Check sheet for the modelled part. Datum: model origin and axes. Units: mm. A direction names the side the tool comes from. Give positions to 0.01 mm unless a question says otherwise; leave off trailing zeros. Loops run counter-clockwise (first coordinate to the right, second up) from the corner with the lowest first, then second, coordinate; pieces in that order, holes last. Notation, with made-up numbers: (47.5, 45) -> (63.5, 45) arc R29 cw to (63.5, 82) -> close; hole circle Ø2 at (-19.5, -28.5). An arc over 180 degrees is marked (long way). Write each question's results on one line, items separated by ' | '. Start each with the question number.
Item 1: Cross-section at D-D on x = -2.5. Enter the section's corners in (y, z), then the cut area to 3 significant figures.
Item 2: Cross-section at A-A on z = 65.5. Enter the section's corners in (x, y).
Item 3: Cross-section at B-B on x = 12.5. Enter the section's corners in (y, z), then the cut area to 3 significant figures.
Item 4: Mould release check, pull along X, two halves, no side actions. Record for faces 1 (the face through (12, -2, 0)), 2 (the face through (10.476, -1.972, 8.448)), 3 (the face through (-16.07, -1.97, 54.5)), 4 (the face through (24, -2, 96)): pulls with the +X half, pulls with the -X half, needs draft (parallel to the pull), parting line crosses it, or undercut.
Item 5: Cross-section at C-C on y = -0.6. Enter the section's corners in (x, z), then the cut area to 3 significant figures.
Item 6: Gauge pin test, flat ends, axial feed: pin 1 Ø6 at (x, z) = (12.5, 10) entering from -Y; pin 2 Ø1 at (y, z) = (-2.5, 29) entering from +X. Record the tip position at first contact, or that the pin passes through.
Item 7: Scan lines: line 1 along Z through (x, y) = (12.5, -2.45); line 2 along X through (y, z) = (-2.8, 67.5); line 3 along Z through (x, y) = (-5.5, -2.6). Record each from-to range of solid material in increasing order.
Item 8: Access from +Z, -Z, +X, -X, +Y, -Y to the whole of each face (thin tool, end or side, straight path). Record for faces 5 (the face through (3, -4, 61)), 6 (the face through (0, -2, 27)).
from build123d import *

# Parameters (mm, degrees)
F0_R     = 2.55
F0_R_2   = 4
F1_DEPTH = 4


with BuildPart() as f1:
    # F0 (on Front) → F1 (new body)
    with BuildSketch(Plane.XZ):
        with BuildLine():
            Line((0, 48), (0, 5))
            ThreePointArc((0, 5), (1.464466, 1.464466), (5, 0))
            Line((5, 0), (20, 0))
            ThreePointArc((20, 0), (21.81842, 0.342388), (23.387798, 1.322661))
            ThreePointArc((23.387798, 1.322661), (16.523699, 23.80604), (25, 45.73252))
            Line((25, 45.73252), (25, 93))
            ThreePointArc((25, 93), (23.535534, 96.535534), (20, 98))
            Line((20, 98), (-12.5, 98))
            ThreePointArc((-12.5, 98), (-16.035534, 96.535534), (-17.5, 93))
            Line((-17.5, 93), (-17.5, 58))
            ThreePointArc((-17.5, 58), (-16.035534, 54.464466), (-12.5, 53))
            Line((-12.5, 53), (-5, 53))
            ThreePointArc((-5, 53), (-1.464466, 51.535534), (0, 48))
        make_face()
        with Locations((12.5, 10)):
            Circle(F0_R, mode=Mode.SUBTRACT)
        with Locations((-2.5, 65.5)):
            Circle(F0_R_2, mode=Mode.SUBTRACT)
        with Locations((12.5, 85.5)):
            Circle(F0_R_2, mode=Mode.SUBTRACT)
    extrude(amount=F1_DEPTH)


solid = f1.part
Answer sheet:
1) outline: (-4, 52.33) -> (0, 52.33) -> (0, 61.5) -> (-4, 61.5) -> close; (-4, 69.5) -> (0, 69.5) -> (0, 98) -> (-4, 98) -> close | area: 151 mm²
2) outline: (-17.5, -4) -> (-6.5, -4) -> (-6.5, 0) -> (-17.5, 0) -> close; (1.5, -4) -> (25, -4) -> (25, 0) -> (1.5, 0) -> close
3) outline: (-4, 0) -> (0, 0) -> (0, 7.45) -> (-4, 7.45) -> close; (-4, 12.55) -> (0, 12.55) -> (0, 81.5) -> (-4, 81.5) -> close; (-4, 89.5) -> (0, 89.5) -> (0, 98) -> (-4, 98) -> close | area: 340 mm²
4) face 1: needs draft | face 2: undercut | face 3: pulls with the -X half | face 4: pulls with the +X half
5) outline: (-17.5, 58) arc R5 ccw to (-12.5, 53) -> (-5, 53) arc R5 cw to (0, 48) -> (0, 5) arc R5 ccw to (5, 0) -> (20, 0) arc R5 ccw to (23.39, 1.32) arc R36 cw to (25, 45.73) -> (25, 93) arc R5 ccw to (20, 98) -> (-12.5, 98) arc R5 ccw to (-17.5, 93) -> close; hole circle Ø8 at (-2.5, 65.5); hole circle Ø8 at (12.5, 85.5); hole circle Ø5.1 at (12.5, 10) | area: 2,830 mm²
6) pin 1: stops at y = -4 | pin 2: stops at x = 17.19
7) line 1: z = 0 to 7.45, 12.55 to 81.5, 89.5 to 98 | line 2: x = -17.5 to -5.96, 0.96 to 25 | line 3: z = 53 to 62.85, 68.15 to 98
8) face 5: +Z, -Z, +X, -X, -Y | face 6: -Z, -X, +Y, -Y
